Part model, mm, in its own coordinate system. A direction names the side the tool comes from. Coordinates: 2 decimals unless noted, no trailing zeros. Write each loop counter-clockwise with the first axis right and the second up, starting at its lowest first coordinate (ties: lowest second). Pieces come first, ordered by that corner, then holes. Notation, with made-up numbers: (61.5, 17.25) - (88.5, 17.25) arc R35 ccw to (88.5, 53.25) - close; hole circle Ø1 at (56.25, -27.75). An arc over 180 degrees is marked (long way). Use a Markdown table: item, result.
```python
from build123d import *

# Parameters (mm, degrees)
SKETCH1_W           = 451
SKETCH1_H           = 490
BOSS_EXTRUDE1_DEPTH = 20
SKETCH2_W           = 429
SKETCH2_H           = 468
CUT_EXTRUDE1_DEPTH  = 18
SKETCH3_W           = 16
SKETCH3_H           = 468
CUT_EXTRUDE2_DEPTH  = 9
SKETCH4_W           = 438
SKETCH4_H           = 16
CUT_EXTRUDE3_DEPTH  = 9
SKETCH5_W           = 16
SKETCH5_H           = 477
CUT_EXTRUDE4_DEPTH  = 9
SKETCH6_W           = 447
SKETCH6_H           = 16
CUT_EXTRUDE5_DEPTH  = 9
FILLET3_R           = 2
FILLET4_R           = 2
SKETCH20_R          = 2.5
CUT_EXTRUDE12_DEPTH = 540.768700463
SKETCH21_R          = 3
CUT_EXTRUDE13_DEPTH = 2
SKETCH22_R          = 3
CUT_EXTRUDE14_DEPTH = 2
SKETCH23_W          = 25
SKETCH23_H          = 100
SKETCH23_W_2        = 6
SKETCH23_H_2        = 22
CUT_EXTRUDE15_DEPTH = 2


with BuildPart() as part:
    # Sketch1 → Boss-Extrude1 (new body)
    with BuildSketch(Plane.XY):
        Rectangle(SKETCH1_W, SKETCH1_H)
    extrude(amount=BOSS_EXTRUDE1_DEPTH)

    # Sketch2 → Cut-Extrude1 (cut)
    with BuildSketch(Plane(origin=(0, 0, 0), x_dir=(-1, 0, 0), z_dir=(0, 0, -1))):
        Rectangle(SKETCH2_W, SKETCH2_H)
    extrude(amount=-CUT_EXTRUDE1_DEPTH, mode=Mode.SUBTRACT)

    # Sketch3 → Cut-Extrude2 (cut)
    with BuildSketch(Plane(origin=(-214.5, 0, 0), x_dir=(0, 0, -1), z_dir=(1, 0, 0))):
        with Locations((-10, 0)):
            Rectangle(SKETCH3_W, SKETCH3_H)
    extrude(amount=-CUT_EXTRUDE2_DEPTH, mode=Mode.SUBTRACT)

    # Sketch4 → Cut-Extrude3 (cut)
    with BuildSketch(Plane(origin=(0, -234, 0), x_dir=(1, 0, 0), z_dir=(0, 1, 0))):
        with Locations((-4.5, -10)):
            Rectangle(SKETCH4_W, SKETCH4_H)
    extrude(amount=-CUT_EXTRUDE3_DEPTH, mode=Mode.SUBTRACT)

    # Sketch5 → Cut-Extrude4 (cut)
    with BuildSketch(Plane.ZY.offset(-214.5)):
        with Locations((10, -4.5)):
            Rectangle(SKETCH5_W, SKETCH5_H)
    extrude(amount=-CUT_EXTRUDE4_DEPTH, mode=Mode.SUBTRACT)

    # Sketch6 → Cut-Extrude5 (cut)
    with BuildSketch(Plane.XZ.offset(-234)):
        with Locations((0, 10)):
            Rectangle(SKETCH6_W, SKETCH6_H)
    extrude(amount=-CUT_EXTRUDE5_DEPTH, mode=Mode.SUBTRACT)

    # Fillet3
    fillet3_edges = [part.edges().sort_by_distance(p)[0] for p in [
        (214.5, 0, 0),
        (225.5, 0, 0),
        (0, 245, 0),
        (0, -245, 0),
        (-225.5, 0, 0),
        (-225.5, 0, 20),
        (0, -245, 20),
        (225.5, 0, 20),
        (0, 245, 20),
    ]]
    fillet(fillet3_edges, radius=FILLET3_R - 0.0001)  # a hair under: the kernel refuses the full size

    # Fillet4
    fillet4_edges = [part.edges().sort_by_distance(p)[0] for p in [
        (0, -243, 18),
        (223.5, 0, 18),
        (0, 243, 18),
        (-223.5, 0, 18),
        (-214.5, 0, 0),
        (0.99995, -234, 0),
        (0.99995, 234, 0),
    ]]
    fillet(fillet4_edges, radius=FILLET4_R - 0.0001)  # a hair under: the kernel refuses the full size

    # Sketch20 → Cut-Extrude12 (cut, through all)
    with BuildSketch(Plane(origin=(0, 245, 0), x_dir=(1, 0, 0), z_dir=(0, 1, 0))):
        with Locations(Location((-217.5, -12, 0), (0, 0, 270))):
            Circle(SKETCH20_R)
    extrude(amount=-CUT_EXTRUDE12_DEPTH, mode=Mode.SUBTRACT)

    # Sketch21 → Cut-Extrude13 (cut)
    with BuildSketch(Plane(origin=(0, 245, 0), x_dir=(1, 0, 0), z_dir=(0, 1, 0))):
        with Locations(Location((187.5, -5, 0), (0, 0, 90))):
            Circle(SKETCH21_R)
    extrude(amount=-CUT_EXTRUDE13_DEPTH, mode=Mode.SUBTRACT)

    # Sketch22 → Cut-Extrude14 (cut)
    with BuildSketch(Plane.XZ.offset(245)):
        with Locations(Location((150.5, 5, 0), (0, 0, 270))):
            Circle(SKETCH22_R)
    extrude(amount=-CUT_EXTRUDE14_DEPTH, mode=Mode.SUBTRACT)

    # Sketch23 → Cut-Extrude15 (cut)
    with BuildSketch(Plane.XY.offset(20)):
        with Locations((169, 0)):
            Rectangle(SKETCH23_W, SKETCH23_H)
        with Locations((198, -86)):
            Rectangle(SKETCH23_W_2, SKETCH23_H_2)
    extrude(amount=-CUT_EXTRUDE15_DEPTH, mode=Mode.SUBTRACT)


solid = part.part
```
Item 1: Band-saw the part on B-B, the plane z = 5. Give the cut face in (x, y), then the cut area to 3 significant figures.
From the geometry:
| item | result |
|---|---|
| outline | (-225.5, -245) - (147.5, -245) - (147.5, -243) - (-223.5, -243) - (-223.5, 243) - (184.5, 243) - (184.5, 245) - (-225.5, 245) - close; (153.5, -245) - (225.5, -245) - (225.5, 245) - (190.5, 245) - (190.5, 243) - (223.5, 243) - (223.5, -243) - (153.5, -243) - close |
| area | 3,720 mm^2 |
Item 2: Two-plate mould, pull along Z, no slides. Class faces 1 (the face through (-216, -109, 2)), 2 (the face through (-3, 3, 20)), 3 (the face through (225.5, -3, 10)): pulls with the +Z half, pulls with the -Z half, needs draft (parallel to the pull), parting line crosses it, or undercut.
From the geometry:
| item | result |
|---|---|
| face 1 | undercut |
| face 2 | pulls with the +Z half |
| face 3 | needs draft |
Item 3: Drop flat-ended pins along their axis: P1, Ø2, axis at x = 23, y = 136.5, coming from the -Z side; P2, Ø0.6, axis at x = 167.5, z = 18.5, coming from the +Y side; P3, Ø0.6, axis at x = 197, z = 19, coming from the +Y side. Give the stop position or say it passes through.
From the geometry:
| item | result |
|---|---|
| P1 | z = 18 |
| P2 | y = 244.99 |
| P3 | y = 244.87 |
Item 4: Which spindle directions (+Z, -Z, +X, -X, +Y, -Y) get a long thin tool onto all of the face, cutting with end or side? Do faces 4 (the face through (-3, -245, 10)), 5 (the face through (-3, -243, 9)). Say none if no direction does.
From the geometry:
| item | result |
|---|---|
| face 4 | +Z, -Z, +X, -X, -Y |
| face 5 | none |
Item 5: Drill centre lines: probe 1 along X at (y, z) = (103.5, 5.25); probe 2 along Y at (x, z) = (42.5, 4.5); probe 3 along X at (y, z) = (243.5, 5). Where is each one in solid material? Low to high.
From the geometry:
| item | result |
|---|---|
| probe 1 | -225.5 to -223.5, 223.5 to 225.5 |
| probe 2 | -245 to -243, 243 to 245 |
| probe 3 | -225.5 to 184.5, 190.5 to 225.5 |
